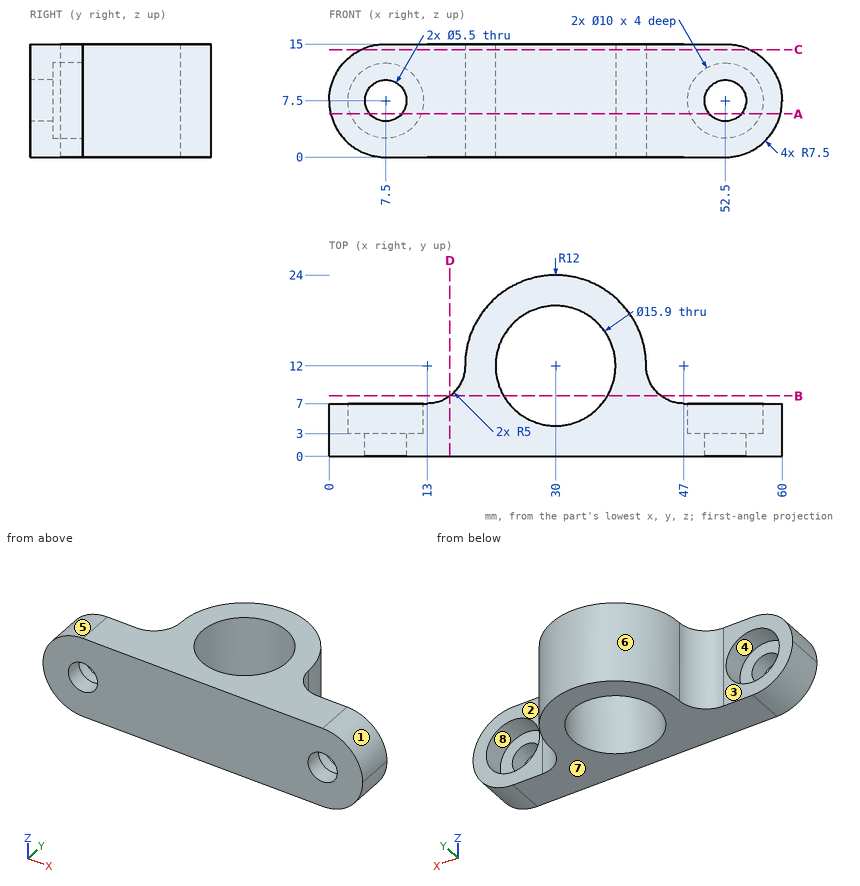
Could you check a few things on this drawing? It's one solid part, dimensions in mm from its lowest x, y, z. A direction names the side the tool comes from. Coordinates: 2 decimals unless noted, no trailing zeros. Order: outer loops, then holes, each group sorted by start corner. A loop starts at its lowest first (then second) coordinate and runs counter-clockwise, first axis right, second up. Notation, with made-up numbers: (-27.75, 19.25) -> (23.25, 19.25) arc R24 ccw to (23.25, 36.25) -> close; hole circle Ø3 at (85, 66). An arc over 180 degrees is marked (long way). One line per item, written item: value. Start each with the question number.
1) I'm going to push flat-ended pins straight in: pin 1 (8 mm diameter, centred on x = 12.5, z = 3, fed in from -Y); pin 2 (8 mm diameter, centred on x = 9, z = 7, fed in from +Y); pin 3 (9 mm diameter, centred on x = 7.5, z = 7.5, fed in from +Y); pin 4 (3 mm diameter, centred on y = 7, z = 4.5, fed in from +X). Where does each tip first touch, or does it pass through?
2) We'd pull the mould along X, two halves only. Please class the marked faces 5, 6, 7 and 8: +X half, -X half, draft (parallel to the pull), parting line (faces both ways), or undercut.
3) Imagine slicing it at D-D on x = 16. List the corners of the cut face in (y, z) for me, plus the area to 3 significant figures.
4) Imagine slicing it at C-C on z = 14.25. List the corners of the cut face in (x, y) for me.
5) If I drill on L1, parallel to X at y = 2.1, z = 7.5; L2, parallel to Y at x = 30, z = 6.5; L3, parallel to Z at x = 52.5, y = 1.65, over which ranges is the centre line in solid material (lowest first)? Write a range as [from, to].
6) Which directions (+Z, -Z, +X, -X, +Y, -Y) give clear straight access to the entire face, cutting with the end or side of a thin tool? Please do the marked faces 1, 2, 3 and 4.
7) Imagine slicing it at B-B on y = 8. List the corners of the cut face in (x, z) for me.
8) Imagine slicing it at A-A on z = 5.75. List the corners of the cut face in (x, y) for me, plus the area to 3 significant figures.
Answer list:
1. pin 1: stops at y = 0
1. pin 2: stops at y = 7
1. pin 3: stops at y = 3
1. pin 4: stops at x = 59.85
2. face 5: -X half
2. face 6: parting line
2. face 7: draft
2. face 8: undercut
3. outline: (0, 0) -> (8, 0) -> (8, 15) -> (0, 15) -> close
3. area: 120 mm2
4. outline: (4.23, 0) -> (55.77, 0) -> (55.77, 7) -> (47, 7) arc R5 cw to (42, 12) arc R12 ccw to (18, 12) arc R5 cw to (13, 7) -> (4.23, 7) -> close; hole circle Ø15.9 at (30, 12)
5. L1: x = [0, 4.75], [10.25, 49.75], [55.25, 60]
5. L2: y = [0, 4.05], [19.95, 24]
5. L3: z = [0, 4.75], [10.25, 15]
6. face 1: +Z, +X, +Y, -Y
6. face 2: +Z, -Z, +X, +Y
6. face 3: +Z, -Z, -X, +Y
6. face 4: +Y
7. outline: (16, 0) -> (23.13, 0) -> (23.13, 15) -> (16, 15) -> close; (36.87, 0) -> (44, 0) -> (44, 15) -> (36.87, 15) -> close
8. outline: (0.21, 0) -> (5.38, 0) -> (5.38, 3) -> (2.82, 3) -> (2.82, 7) -> (0.21, 7) -> close; (9.62, 0) -> (50.38, 0) -> (50.38, 3) -> (47.82, 3) -> (47.82, 7) -> (47, 7) arc R5 cw to (42, 12) arc R12 ccw to (18, 12) arc R5 cw to (13, 7) -> (12.18, 7) -> (12.18, 3) -> (9.62, 3) -> close; (54.62, 0) -> (59.79, 0) -> (59.79, 7) -> (57.18, 7) -> (57.18, 3) -> (54.62, 3) -> close; hole circle Ø15.9 at (30, 12)
8. area: 475 mm2
